Verification items for the finished model (mm, model axes). A direction names the side the tool comes from. Round coordinates to 2 decimals unless told otherwise and drop trailing zeros. Order: outer loops, then holes, each group sorted by start corner. A loop starts at its lowest first (then second) coordinate and runs counter-clockwise, first axis right, second up. Notation, with made-up numbers: (26.5, 39) -> (69.5, 39) arc R7 cw to (69.5, 43) -> close; hole circle Ø10 at (67, -15.5). An arc over 180 degrees is marked (long way). Put each result on its own line as item: value.
```python
from build123d import *

# Parameters (mm, degrees)
PAD_DEPTH   = 40
FILLET_R    = 75
FILLET001_R = 5
FILLET002_R = 1
FILLET003_R = 3
FILLET004_R = 1


with BuildPart() as part:
    # Sketch → Pad (new body)
    with BuildSketch(Plane.XY):
        Polygon((-94, 182), (-117, 182), (-117, 165.515676), (-90.103703, 0), (90.103703, 0), (117, 165.515676), (117, 182), (94, 182), (94, 176), (111, 176), (111, 166), (85, 6), (-85, 6), (-111, 166), (-111, 176), (-94, 176), align=None)
    extrude(amount=PAD_DEPTH)

    # Fillet
    fillet_edges = [part.edges().sort_by_distance(p)[0] for p in [
        (117, 165.515676, 20),
        (-117, 165.515676, 20),
        (111, 166, 20),
        (-111, 166, 20),
    ]]
    fillet(fillet_edges, radius=FILLET_R)

    # Fillet001
    fillet001_edges = [part.edges().sort_by_distance(p)[0] for p in [
        (-90.103703, 0, 20),
        (90.103703, 0, 20),
    ]]
    fillet(fillet001_edges, radius=FILLET001_R)

    # Fillet002
    fillet002_edges = [part.edges().sort_by_distance(p)[0] for p in [
        (85, 6, 20),
        (-85, 6, 20),
    ]]
    fillet(fillet002_edges, radius=FILLET002_R)

    # Fillet003
    fillet003_edges = [part.edges().sort_by_distance(p)[0] for p in [
        (117, 182, 20),
        (-117, 182, 20),
        (-94, 182, 20),
        (94, 182, 20),
    ]]
    fillet(fillet003_edges, radius=FILLET003_R)

    # Fillet004
    fillet004_edges = [part.edges().sort_by_distance(p)[0] for p in [
        (-94, 176, 20),
        (-111, 176, 20),
        (111, 176, 20),
        (94, 176, 20),
    ]]
    fillet(fillet004_edges, radius=FILLET004_R)


solid = part.part
```
Item 1: Material ranges on line 1 along X through (y, z) = (171, 33); line 2 along Y through (x, z) = (35, 7); line 3 along X through (y, z) = (135.5, 22), recorded low to high.
Geometry check:
line 1: -117 to -110.99, 110.99 to 117
line 2: 0 to 6
line 3: -112.12 to -106.04, 106.04 to 112.12
Item 2: Sectioned sample at C-C, the plane x = 39. Record the boundary of the cut face in (y, z).
Geometry check:
outline: (0, 0) -> (6, 0) -> (6, 40) -> (0, 40) -> close
Item 3: Tool access check on faces 5 (the face through (1, 6, 20)), 6 (the face through (102, 176, 20)), 7 (the face through (116.75, 165.45, 20.28)). Record the directions out of +Z, -Z, +X, -X, +Y, -Y that give a thin tool (end or side, any length) a straight path to the whole face; none if there is none.
Geometry check:
face 5: +Z, -Z, +Y
face 6: +Z, -Z
face 7: +Z, -Z, +X, -Y
Item 4: Depth check by flat-ended pin: pin 1 Ø20 at (x, z) = (-14, 28.5) entering from +Y; pin 2 Ø1.5 at (y, z) = (143.5, 21) entering from +X; pin 3 Ø6 at (y, z) = (116, 26) entering from +X. Enter the tip coordinate at first touch or a pass-through.
Geometry check:
pin 1: y = 6
pin 2: x = 113.54
pin 3: x = 109.44
Item 5: Sectioned sample at B-B, the plane y = 45.5. Record the boundary of the cut face in (x, z).
Geometry check:
outline: (-97.5, 0) -> (-91.42, 0) -> (-91.42, 40) -> (-97.5, 40) -> close; (91.42, 0) -> (97.5, 0) -> (97.5, 40) -> (91.42, 40) -> close
Item 6: Release check for a two-part mould opening along Y. For faces 1 (the face through (-97.41, 82.36, 19.72)), 2 (the face through (117, 175, 20)), 3 (the face through (103.23, 80.78, 19.72)), 4 (the face through (97.757, 84.504, 19.72)) record: pulls with the +Y half, pulls with the -Y half, needs draft (parallel to the pull), parting line crosses it, or undercut.
Geometry check:
face 1: undercut
face 2: needs draft
face 3: pulls with the -Y half
face 4: undercut
